Here's how the part is built. I have some questions about the finished solid (model axes, mm). Round coordinates to 2 decimals unless told otherwise and drop trailing zeros. Order: outer loops, then holes, each group sorted by start corner. A loop starts at its lowest first (then second) coordinate and runs counter-clockwise, first axis right, second up. Notation, with made-up numbers: (35.25, 54.25) -> (69.25, 54.25) arc R14 ccw to (69.25, 75.25) -> close; hole circle Ø4 at (40.25, 41.5). An arc over 180 degrees is marked (long way). Use a Markdown table: item, result. Add a question column.
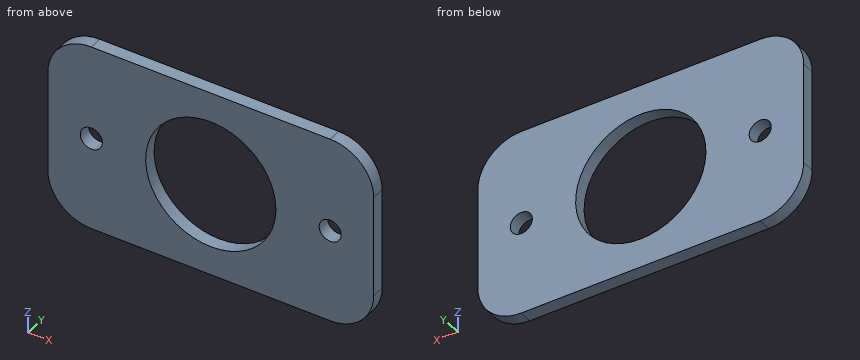
from build123d import *

# Parameters (mm, degrees)
SKETCH_1_W             = 75
SKETCH_1_H             = 43.638217254
SM_BASE_FLANGE_1_DEPTH = 3
SKETCH_8_R             = 15
CUT_EXTRUDE_1_DEPTH    = 74.36050648
FILLET_1_R             = 10
SKETCH_9_R             = 2.54
CUT_EXTRUDE_2_DEPTH    = 10


# Sheet-metal steps are written as plain solids
with BuildPart() as part:
    # Sketch 1 → 基体-法兰1 (new body)
    with BuildSketch(Plane(origin=(0, 0, 0), x_dir=(1, 0, 0), z_dir=(0, 1, 0))):
        with Locations((27.582223351, 11.901331978)):
            Rectangle(SKETCH_1_W, SKETCH_1_H)
    extrude(amount=-SM_BASE_FLANGE_1_DEPTH)

    # 草图8 → 切除-拉伸1 (cut, through all)
    with BuildSketch(Plane(origin=(0, -3, 0), x_dir=(-1, 0, 0), z_dir=(0, -1, 0))):
        with Locations(Location((-27.582223351, 12, 0), (0, 0, 90))):
            Circle(SKETCH_8_R)
    extrude(amount=-CUT_EXTRUDE_1_DEPTH, mode=Mode.SUBTRACT)

    # 圆角1
    fillet_1_edges = [part.edges().sort_by_distance(p)[0] for p in [
        (65.082223351, -1.5, 9.917776649),
        (-9.917776649, -1.5, 9.917776649),
        (-9.917776649, -1.5, -33.720440605),
        (65.082223351, -1.5, -33.720440605),
    ]]
    fillet(fillet_1_edges, radius=FILLET_1_R)

    # 草图9 → 切除-拉伸2 (cut)
    with BuildSketch(Plane(origin=(0, 0, 0), x_dir=(1, 0, 0), z_dir=(0, 1, 0))):
        with Locations(Location((0.082223351, 12.082223351, 0), (0, 0, 270))):
            Circle(SKETCH_9_R)
        with Locations(Location((55.082223351, 12.082223351, 0), (0, 0, 270))):
            Circle(SKETCH_9_R)
    extrude(amount=-CUT_EXTRUDE_2_DEPTH, mode=Mode.SUBTRACT)


solid = part.part
(1) Please list where these lines run through material, in increasing order: probe 1 along X at (y, z) = (-2.25, -11.5); probe 2 along X at (y, z) = (-0.25, -11); probe 3 along Z at (x, y) = (-0.5, -0.6). Write a range as from..to.
(2) I want a section at C-C on y = -0.6. List the corners of the cut face in (x, z) for me, and give its area (3 significant figures).
(3) I want a section at A-A on x = 22. List the corners of the cut face in (y, z) for me.
(4) I want a section at D-D on z = -21. List the corners of the cut face in (x, y) for me.
(5) I want a section at B-B on z = -12. List the corners of the cut face in (x, y) for me.
(6) I'm going to push a flat-ended pin straight in: P1, Ø1.5, axis at y = -2, z = -24, coming from the -X side. Where does the tip first touch, or does it pass through?
Output:
| question | item | result |
|---|---|---|
| 1 | probe 1 | -9.92..-2.39, 2.55..12.59, 42.57..52.61, 57.55..65.08 |
| 1 | probe 2 | -9.92..-2.22, 2.38..12.62, 42.55..52.78, 57.38..65.08 |
| 1 | probe 3 | -33.7..-14.55, -9.61..9.9 |
| 2 | outline | (-9.92, -23.72) arc R10 ccw to (0.08, -33.72) -> (55.08, -33.72) arc R10 ccw to (65.08, -23.72) -> (65.08, -0.08) arc R10 ccw to (55.08, 9.92) -> (0.08, 9.92) arc R10 ccw to (-9.92, -0.08) -> close; hole circle Ø5.08 at (0.08, -12.08); hole circle Ø30 at (27.58, -12); hole circle Ø5.08 at (55.08, -12.08) |
| 2 | area | 2,440 mm² |
| 3 | outline | (-3, -33.72) -> (0, -33.72) -> (0, -25.92) -> (-3, -25.92) -> close; (-3, 1.92) -> (0, 1.92) -> (0, 9.92) -> (-3, 9.92) -> close |
| 4 | outline | (-9.92, -3) -> (15.58, -3) -> (15.58, 0) -> (-9.92, 0) -> close; (39.58, -3) -> (65.08, -3) -> (65.08, 0) -> (39.58, 0) -> close |
| 5 | outline | (-9.92, -3) -> (-2.46, -3) -> (-2.46, 0) -> (-9.92, 0) -> close; (2.62, -3) -> (12.58, -3) -> (12.58, 0) -> (2.62, 0) -> close; (42.58, -3) -> (52.54, -3) -> (52.54, 0) -> (42.58, 0) -> close; (57.62, -3) -> (65.08, -3) -> (65.08, 0) -> (57.62, 0) -> close |
| 6 | P1 | x = -9.92 |
